Read the model definition and answer for the solid it produces. Units are mm, in the model's axes. Face numbers are marked on the shaded views. A direction names the side the tool comes from. Coordinates: 2 decimals unless noted, no trailing zeros. Loops run counter-clockwise (first coordinate to the right, second up) from the corner with the lowest first, then second, coordinate; pieces in that order, holes last. Notation, with made-up numbers: M 34.5,73 L 38.5,73 A36 cw 38.5,110 Z; hole C 7,-9 d1. An arc over 180 degrees is marked long. One line per item, written item: value. Start each with the question number.
```python
from build123d import *

# Parameters (mm, degrees)
F0_W      = 63.5
F0_H      = 25.4
F0_W_2    = 58.42
F0_H_2    = 20.32
F1_DEPTH  = 50.8
F2_W      = 58.42
F2_H      = 20.32
F3_DEPTH  = 2.54
F4_R      = 10.16
F5_DEPTH  = 63.501
F7_W      = 12.7
F7_H      = 1.5
F8_DEPTH  = 7.62
F10_R     = 1.5
F11_DEPTH = 25.4
F12_R     = 1.5
F13_DEPTH = 25.4
F14_R     = 5.08
F6_W      = 24.13
F6_H      = 12.954
F15_DEPTH = 25.4


with BuildPart() as f1:
    # F0 (on Top) → F1 (new body)
    with BuildSketch(Plane.XY):
        Rectangle(F0_W, F0_H)
        Rectangle(F0_W_2, F0_H_2, mode=Mode.SUBTRACT)
    extrude(amount=F1_DEPTH)

    # F2 (on face) → F3 (join)
    with BuildSketch(Plane(origin=(0, 0, 0), x_dir=(1, 0, 0), z_dir=(0, 0, -1))):
        Rectangle(F2_W, F2_H)
    extrude(amount=-F3_DEPTH)

    # F4 (on face) → F5 (cut, through all)
    with BuildSketch(Plane(origin=(-31.75, 0, 0), x_dir=(0, -1, 0), z_dir=(-1, 0, 0))):
        with Locations((0, 50.8)):
            Circle(F4_R)
    extrude(amount=-F5_DEPTH, mode=Mode.SUBTRACT)

    # F7 (on face) → F8 (join)
    with BuildSketch(Plane.XZ.offset(12.7)):
        with Locations((0, 50.05)):
            Rectangle(F7_W, F7_H)
    extrude(amount=F8_DEPTH)

    # F9: F1 across plane


with BuildPart() as f1_1:
    add(f1.part)
    add(f1.part.mirror(Plane.XZ))

    # F10 (on face) → F11 (cut)
    with BuildSketch(Plane.XY.offset(50.8)):
        with Locations((0, -16.51)):
            Circle(F10_R)
    extrude(amount=-F11_DEPTH, mode=Mode.SUBTRACT)

    # F12 (on face) → F13 (cut)
    with BuildSketch(Plane(origin=(0, 0, 49.3), x_dir=(1, 0, 0), z_dir=(0, 0, -1))):
        with Locations((0, -16.51)):
            Circle(F12_R)
    extrude(amount=-F13_DEPTH, mode=Mode.SUBTRACT)

    # F14
    f14_edges = [f1_1.edges().sort_by_distance(p)[0] for p in [
        (6.35, 20.32, 50.05),
        (-6.35, 20.32, 50.05),
        (6.35, -20.32, 50.05),
        (-6.35, -20.32, 50.05),
    ]]
    fillet(f14_edges, radius=F14_R)

    # F6 (on face) → F15 (cut)
    with BuildSketch(Plane(origin=(0, 0, 0), x_dir=(1, 0, 0), z_dir=(0, 0, -1))):
        Rectangle(F6_W, F6_H)
    extrude(amount=-F15_DEPTH, mode=Mode.SUBTRACT)


solid = f1_1.part
```
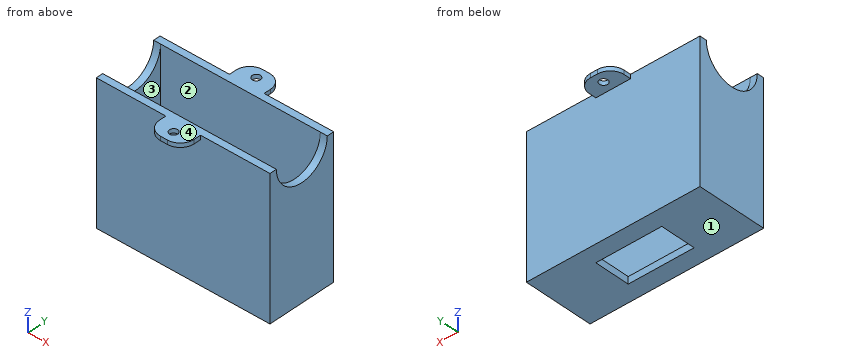
1) Section D-D (x = 0) is taken. Determine the outline of the cut face in (y, z), then the cut area to 3 significant figures.
2) Section B-B (y = 0) is taken. Determine the outline of the cut face in (x, z) (3 decimals), then the cut area to 3 significant figures.
3) Consider line 1 along Y through (x, z) = (0, 49.85); line 2 along Y through (x, z) = (3, 21.5); line 3 along Z through (x, y) = (0.5, -10). Determine where each line is inside the solid, lowest interval first.
4) Section A-A (x = -8) is taken. Determine the outline of the cut face in (y, z).
5) Section C-C (z = 18) is taken. Determine the outline of the cut face in (x, y).
6) A tool of negligible diameter and unlimited length cuts with its end or side. For the marked faces 1 and 2, from which of +Z, -Z, +X, -X, +Y, -Y can it reach the whole face along a straight path? Write none if from no direction.
7) Flat-ended cylindrical pins translate along their axes: pin 1 (10 mm diameter, centred on x = 15.5, z = 45.5, fed in from -Y); pin 2 (1.2 mm diameter, centred on y = -14, z = 50, fed in from -X); pin 3 (22.5 mm diameter, centred on x = 0, y = -1, fed in from +Z); pin 4 (6 mm diameter, centred on x = 2.5, y = -17, fed in from -Z). Find the tip coordinate at first contact, or state that the pin passes through.
8) For a pull along Y with two mould halves and no side action, classify the marked faces 3 and 4 as released by +Y, released by -Y, zero draft, split by the parting line, or undercut.
Results found:
1. outline: M -20.32,49.3 L -18.01,49.3 L -18.01,50.8 L -20.32,50.8 Z; M -15.01,49.3 L -12.7,49.3 L -12.7,0 L -6.48,0 L -6.48,2.54 L -10.16,2.54 L -10.16,50.8 L -15.01,50.8 Z; M 6.48,0 L 12.7,0 L 12.7,49.3 L 15.01,49.3 L 15.01,50.8 L 10.16,50.8 L 10.16,2.54 L 6.48,2.54 Z; M 18.01,49.3 L 20.32,49.3 L 20.32,50.8 L 18.01,50.8 Z
1. area: 291 mm²
2. outline: M -31.75,0 L -12.065,0 L -12.065,2.54 L -29.21,2.54 L -29.21,40.64 L -31.75,40.64 Z; M 12.065,0 L 31.75,0 L 31.75,40.64 L 29.21,40.64 L 29.21,2.54 L 12.065,2.54 Z
2. area: 294 mm²
3. line 1: y = -20.32 to -18.01, -15.01 to -10.16, 10.16 to 15.01, 18.01 to 20.32
3. line 2: y = -12.7 to -10.16, 10.16 to 12.7
3. line 3: z = 0 to 2.54
4. outline: M -12.7,0 L -6.48,0 L -6.48,2.54 L -10.16,2.54 L -10.16,50.8 L -12.7,50.8 Z; M 6.48,0 L 12.7,0 L 12.7,50.8 L 10.16,50.8 L 10.16,2.54 L 6.48,2.54 Z
5. outline: M -31.75,-12.7 L 31.75,-12.7 L 31.75,12.7 L -31.75,12.7 Z; hole M -29.21,-10.16 L 29.21,-10.16 L 29.21,10.16 L -29.21,10.16 Z
6. face 1: -Z, +X, -X, +Y, -Y
6. face 2: +Z
7. pin 1: stops at y = -12.7
7. pin 2: stops at x = -6.35
7. pin 3: stops at z = 50.8
7. pin 4: stops at z = 49.3
8. face 3: undercut
8. face 4: zero draft
